Geometry check sheet. Reference: the model listing, model coordinates, mm. Give positions to 0.01 mm unless a question says otherwise; leave off trailing zeros. Write each loop counter-clockwise with the first axis right and the second up, starting at its lowest first coordinate (ties: lowest second). Pieces come first, ordered by that corner, then holes. Notation, with made-up numbers: M 74.5,49 L 124.5,49 A27 ccw 124.5,70 Z; hole C 45.5,-11 d7. An arc over 180 degrees is marked long. One line per item, written item: value. Start each with the question number.
1. Cross-section at B-B on z = 4.25. Record the cut outline in (x, y) (1 decimal).
2. Release check for a two-part mould opening along X. For faces 1 (the face through (0, -11, 0)), 2 (the face through (1.72, 7.75, 2.35)), 3 (the face through (-0.24, 11.11, 2.35)), 4 (the face through (13.965, -12.263, 2.348)) record: pulls with the +X half, pulls with the -X half, needs draft (parallel to the pull), parting line crosses it, or undercut.
3. Scan lines: line 1 (Y direction, x = 0, z = 3.1); line 2 (Y direction, x = -3, z = 1.4); line 3 (X direction, y = 7, z = 3.4). Record each from-to range of solid material in increasing order.
4. Cross-section at D-D on y = -13. Record the cut outline in (x, z).
5. Cross-section at A-A on x = 0. Record the cut outline in (y, z), then the cut area to 3 significant figures.
6. Gauge pin test, flat ends, axial feed: pin 1 (1.5 mm diameter, centred on x = -10.5, z = 1.5, fed in from +Y); pin 2 (1 mm diameter, centred on y = -19.5, z = 2, fed in from -X). Record the tip position at first contact, or that the pin passes through.
7. Cross-section at C-C on y = 4. Record the cut outline in (x, z), then the cut area to 3 significant figures.
from build123d import *

# Parameters (mm, degrees)
SKETCH1_R           = 7.9375
BOSS_EXTRUDE1_DEPTH = 4.7625


with BuildPart() as part:
    # Sketch1 → Boss-Extrude1 (new body)
    with BuildSketch(Plane.XY):
        with BuildLine():
            ThreePointArc((11.1125, 0), (14.0454446, -12.4241527), (22.225, -22.225))
            Line((22.225, -22.225), (22.225, -25.4))
            Line((22.225, -25.4), (-22.225, -25.4))
            Line((-22.225, -25.4), (-22.225, -22.225))
            ThreePointArc((-22.225, -22.225), (-14.0454446, -12.4241527), (-11.1125, 0))
            ThreePointArc((-11.1125, 0), (0, 11.1125), (11.1125, 0))
        make_face()
        with Locations(Location((0, 0, 0), (0, 0, 180))):
            Circle(SKETCH1_R, mode=Mode.SUBTRACT)
    extrude(amount=BOSS_EXTRUDE1_DEPTH)


solid = part.part
Report:
1. outline: M -22.2,-25.4 L 22.2,-25.4 L 22.2,-22.2 A27.8 cw 11.1,0 A11.1 ccw -11.1,0 A27.8 cw -22.2,-22.2 Z; hole C 0,0 d15.9
2. face 1: needs draft
2. face 2: undercut
2. face 3: parting line crosses it
2. face 4: pulls with the +X half
3. line 1: y = -25.4 to -7.94, 7.94 to 11.11
3. line 2: y = -25.4 to -7.35, 7.35 to 10.7
3. line 3: x = -8.63 to -3.74, 3.74 to 8.63
4. outline: M -14.34,0 L 14.34,0 L 14.34,4.76 L -14.34,4.76 Z
5. outline: M -25.4,0 L -7.94,0 L -7.94,4.76 L -25.4,4.76 Z; M 7.94,0 L 11.11,0 L 11.11,4.76 L 7.94,4.76 Z
5. area: 98.3 mm^2
6. pin 1: stops at y = 5.33
6. pin 2: stops at x = -19.61
7. outline: M -10.37,0 L -6.86,0 L -6.86,4.76 L -10.37,4.76 Z; M 6.86,0 L 10.37,0 L 10.37,4.76 L 6.86,4.76 Z
7. area: 33.4 mm^2
